from build123d import *

# Parameters (mm, degrees)
SKETCH1_R           = 1.5
SKETCH1_W           = 166
SKETCH1_H           = 3
SKETCH1_H_2         = 62
SKETCH1_W_2         = 70
SKETCH1_H_3         = 174.5
BOSS_EXTRUDE1_DEPTH = 6
FILLET_1_R          = 10


with BuildPart() as part:
    # Sketch1 → Boss-Extrude1 (new body)
    with BuildSketch(Plane(origin=(0, 0, 0), x_dir=(1, 0, 0), z_dir=(0, 1, 0))):
        with BuildLine():
            Line((216, -40), (216, -255))
            ThreePointArc((216, -255), (233, -272), (250, -255))
            Line((250, -255), (250, 0))
            Line((250, 0), (253, 0))
            Line((253, 0), (253, 50))
            Line((253, 50), (250, 50))
            Line((250, 50), (250, 259.060301809))
            ThreePointArc((250, 259.060301809), (233, 276.060301809), (216, 259.060301809))
            Line((216, 259.060301809), (216, 91.5))
            Line((216, 91.5), (50, 91.5))
            Line((50, 91.5), (50, 150))
            Line((50, 150), (-60, 150))
            Line((-60, 150), (-60, 91.5))
            Line((-60, 91.5), (-226, 91.5))
            Line((-226, 91.5), (-226, 259.060301809))
            ThreePointArc((-226, 259.060301809), (-243, 276.060301809), (-260, 259.060301809))
            Line((-260, 259.060301809), (-260, 50))
            Line((-260, 50), (-263, 50))
            Line((-263, 50), (-263, 0))
            Line((-263, 0), (-260, 0))
            Line((-260, 0), (-260, -255))
            ThreePointArc((-260, -255), (-243, -272), (-226, -255))
            Line((-226, -255), (-226, -40))
            Line((-226, -40), (-202.5, -16.5))
            Line((-202.5, -16.5), (-60, -16.5))
            Line((-60, -16.5), (-60, -120))
            Line((-60, -120), (50, -120))
            Line((50, -120), (50, -16.5))
            Line((50, -16.5), (192.5, -16.5))
            Line((192.5, -16.5), (216, -40))
        make_face()
        with Locations(Location((238.092169369, 265.230375643, 0), (0, 0, 270))):
            Circle(SKETCH1_R, mode=Mode.SUBTRACT)
        with Locations(Location((225.673037322, 265.107252935, 0), (0, 0, 270))):
            Circle(SKETCH1_R, mode=Mode.SUBTRACT)
        with Locations(Location((227.907830631, 252.890227975, 0), (0, 0, 270))):
            Circle(SKETCH1_R, mode=Mode.SUBTRACT)
        with Locations(Location((240.326962678, 253.013350683, 0), (0, 0, 270))):
            Circle(SKETCH1_R, mode=Mode.SUBTRACT)
        with Locations(Location((226.282485579, -248.282485579, 0), (0, 0, 270))):
            Circle(SKETCH1_R, mode=Mode.SUBTRACT)
        with Locations(Location((238.656854249, -249.343145751, 0), (0, 0, 270))):
            Circle(SKETCH1_R, mode=Mode.SUBTRACT)
        with Locations(Location((239.717514421, -261.717514421, 0), (0, 0, 270))):
            Circle(SKETCH1_R, mode=Mode.SUBTRACT)
        with Locations(Location((227.343145751, -260.656854249, 0), (0, 0, 270))):
            Circle(SKETCH1_R, mode=Mode.SUBTRACT)
        with Locations(Location((22.5, 125, 0), (0, 0, 270))):
            Circle(SKETCH1_R, mode=Mode.SUBTRACT)
        with Locations(Location((-32.5, 125, 0), (0, 0, 270))):
            Circle(SKETCH1_R, mode=Mode.SUBTRACT)
        with Locations(Location((-237.343145751, -260.656854249, 0), (0, 0, 270))):
            Circle(SKETCH1_R, mode=Mode.SUBTRACT)
        with Locations(Location((-249.717514421, -261.717514421, 0), (0, 0, 270))):
            Circle(SKETCH1_R, mode=Mode.SUBTRACT)
        with Locations(Location((-248.656854249, -249.343145751, 0), (0, 0, 270))):
            Circle(SKETCH1_R, mode=Mode.SUBTRACT)
        with Locations(Location((-236.282485579, -248.282485579, 0), (0, 0, 270))):
            Circle(SKETCH1_R, mode=Mode.SUBTRACT)
        with Locations(Location((-250.326962678, 253.013350683, 0), (0, 0, 270))):
            Circle(SKETCH1_R, mode=Mode.SUBTRACT)
        with Locations(Location((-237.907830631, 252.890227975, 0), (0, 0, 270))):
            Circle(SKETCH1_R, mode=Mode.SUBTRACT)
        with Locations(Location((-235.673037322, 265.107252935, 0), (0, 0, 270))):
            Circle(SKETCH1_R, mode=Mode.SUBTRACT)
        with Locations(Location((-248.092169369, 265.230375643, 0), (0, 0, 270))):
            Circle(SKETCH1_R, mode=Mode.SUBTRACT)
        with Locations(Location((22.5, -92.5, 0), (0, 0, 270))):
            Circle(SKETCH1_R, mode=Mode.SUBTRACT)
        with Locations(Location((-32.5, -92.5, 0), (0, 0, 270))):
            Circle(SKETCH1_R, mode=Mode.SUBTRACT)
        with Locations((133, 80)):
            Rectangle(SKETCH1_W, SKETCH1_H, mode=Mode.SUBTRACT)
        with Locations((133, 37.5)):
            Rectangle(SKETCH1_W, SKETCH1_H_2, mode=Mode.SUBTRACT)
        with Locations((-143, 37.5)):
            Rectangle(SKETCH1_W, SKETCH1_H_2, mode=Mode.SUBTRACT)
        with Locations((133, -5)):
            Rectangle(SKETCH1_W, SKETCH1_H, mode=Mode.SUBTRACT)
        with Locations((-143, -5)):
            Rectangle(SKETCH1_W, SKETCH1_H, mode=Mode.SUBTRACT)
        with Locations((-143, 80)):
            Rectangle(SKETCH1_W, SKETCH1_H, mode=Mode.SUBTRACT)
        with Locations((-5, 16.25)):
            Rectangle(SKETCH1_W_2, SKETCH1_H_3, mode=Mode.SUBTRACT)
    extrude(amount=BOSS_EXTRUDE1_DEPTH)

    # Скругление1
    fillet_1_edges = [part.edges().sort_by_distance(p)[0] for p in [
        (30, 3, 71),
        (30, 3, -103.5),
        (-40, 3, -103.5),
        (-40, 3, 71),
        (216, 3, -6.5),
        (216, 3, -68.5),
        (50, 3, -68.5),
        (50, 3, -6.5),
        (-226, 3, -68.5),
        (-226, 3, -6.5),
        (-60, 3, -6.5),
        (-60, 3, -68.5),
        (-226, 3, -91.5),
        (-60, 3, -91.5),
        (-60, 3, -150),
        (50, 3, -150),
        (50, 3, -91.5),
        (216, 3, -91.5),
        (216, 3, 40),
        (192.5, 3, 16.5),
        (50, 3, 16.5),
        (50, 3, 120),
        (-60, 3, 120),
        (-60, 3, 16.5),
        (-202.5, 3, 16.5),
        (-226, 3, 40),
    ]]
    fillet(fillet_1_edges, radius=FILLET_1_R)


solid = part.part
For this review, take the finished solid that the model builds, in its own axes (mm). A direction names the side the tool comes from. Round coordinates to 2 decimals unless told otherwise and drop trailing zeros. Loops run counter-clockwise (first coordinate to the right, second up) from the corner with the lowest first, then second, coordinate; pieces in that order, holes last. Notation, with made-up numbers: (78, 37.5) - (111, 37.5) arc R22 ccw to (111, 58.5) - close; hole circle Ø9 at (53, -11.75). An arc over 180 degrees is marked (long way). One line per item, written item: value. Start each with the question number.
Item 1: Take a section at C-C (z = 173). Give the boundary of the cut face in (x, y).
Item 2: Take a section at B-B (x = -147). Give the boundary of the cut face in (y, z).
Item 3: Take a section at D-D (y = 2.75). State how many separate pieces and enclosed holes the cut face has, plus the area to 3 significant figures.
Item 4: The part is to be moulded in two halves that separate along X. For faces 1 (the flat face through (-44, 0, -3)), 2 (the cylindrical face through (233, 3, 272)), say which applies: +X half, -X half, draft (parallel to the pull), parting line (faces both ways), or undercut.
Item 5: Clearance check with flat-ended pins moving along their axes: pin 1 Ø1.5 at (x, y) = (-85, 1.5) entering from -Z; pin 2 Ø3.5 at (y, z) = (4, -79.5) entering from -X; pin 3 Ø3 at (y, z) = (4, 85) entering from +X; pin 4 Ø2.5 at (x, z) = (22.5, 92.5) entering from -Y. State where each tip first meets the part, or that it passes through.
Item 6: For L1, parallel to X at y = 3.6, z = 89; L2, parallel to Z at x = -81, y = 3.5; L3, parallel to X at y = 3.6, z = -80.5, list the stretches that pass through material, from the lowest coordinate up.
Item 7: Take a section at A-A (z = 51). Give the boundary of the cut face in (x, y), plus the area to 3 significant figures.
Item 8: For faces 3 (the flat face through (-214, 3, 28)), 4 (the flat face through (-44, 6, -3)), list the 3-axis set-ups (+Z, -Z, +X, -X, +Y, -Y) from which the entire face can be reached by the end or side of a thin tool; tool diameter is ignored.
Answer below:
1. outline: (-260, 0) - (-226, 0) - (-226, 6) - (-260, 6) - close; (216, 0) - (250, 0) - (250, 6) - (216, 6) - close
2. outline: (0, -91.5) - (6, -91.5) - (6, -81.5) - (0, -81.5) - close; (0, -78.5) - (6, -78.5) - (6, -68.5) - (0, -68.5) - close; (0, -6.5) - (6, -6.5) - (6, 3.5) - (0, 3.5) - close; (0, 6.5) - (6, 6.5) - (6, 16.5) - (0, 16.5) - close
3. separate pieces: 1
3. enclosed holes: 27
3. area: 68,600 mm2
4. face 1: draft
4. face 2: undercut
5. pin 1: stops at z = -91.5
5. pin 2: stops at x = -260
5. pin 3: stops at x = 250
5. pin 4: passes through
6. L1: x = -260 to -226, -60 to 50, 216 to 250
6. L2: z = -91.5 to -81.5, -78.5 to -68.5, -6.5 to 3.5, 6.5 to 16.5
6. L3: x = -260 to -226, -60 to -40, 30 to 50, 216 to 250
7. outline: (-260, 0) - (-226, 0) - (-226, 6) - (-260, 6) - close; (-60, 0) - (-40, 0) - (-40, 6) - (-60, 6) - close; (30, 0) - (50, 0) - (50, 6) - (30, 6) - close; (216, 0) - (250, 0) - (250, 6) - (216, 6) - close
7. area: 648 mm2
8. face 3: +Z, +Y, -Y
8. face 4: +Z, -Z, +X, -X, +Y
